from build123d import *

# Parameters (mm, degrees)
CROQUIS1_W              = 111
CROQUIS1_H              = 40
SALIENTE_EXTRUIR1_DEPTH = 5
CROQUIS2_R              = 2
CROQUIS2_W              = 52.7
CROQUIS2_H              = 11.179597985
CORTAR_EXTRUIR1_DEPTH   = 10
CROQUIS3_W              = 5
CROQUIS3_H              = 13.3
SALIENTE_EXTRUIR2_DEPTH = 5
CROQUIS4_W              = 5
CROQUIS4_H              = 13.3
SALIENTE_EXTRUIR3_DEPTH = 5


with BuildPart() as part:
    # Croquis1 → Saliente-Extruir1 (new body)
    with BuildSketch(Plane.XY):
        with Locations((55.5, 20)):
            Rectangle(CROQUIS1_W, CROQUIS1_H)
    extrude(amount=SALIENTE_EXTRUIR1_DEPTH)

    # Croquis2 → Cortar-Extruir1 (cut)
    with BuildSketch(Plane.XY.offset(5)):
        with Locations((24.25, 24.5)):
            Circle(CROQUIS2_R)
        with Locations((86.75, 24.5)):
            Circle(CROQUIS2_R)
        with Locations((24.25, 4.9)):
            Circle(CROQUIS2_R)
        with Locations((86.75, 4.9)):
            Circle(CROQUIS2_R)
        with Locations((54.905498666, 24.410201008)):
            Rectangle(CROQUIS2_W, CROQUIS2_H)
    extrude(amount=-CORTAR_EXTRUIR1_DEPTH, mode=Mode.SUBTRACT)

    # Croquis3 → Saliente-Extruir2 (add)
    with BuildSketch(Plane.ZY):
        with Locations((2.5, 17.85)):
            Rectangle(CROQUIS3_W, CROQUIS3_H)
    extrude(amount=SALIENTE_EXTRUIR2_DEPTH)

    # Croquis4 → Saliente-Extruir3 (add)
    with BuildSketch(Plane(origin=(111, 0, 0), x_dir=(0, 0, -1), z_dir=(1, 0, 0))):
        with Locations((-2.5, 17.85)):
            Rectangle(CROQUIS4_W, CROQUIS4_H)
    extrude(amount=SALIENTE_EXTRUIR3_DEPTH)


solid = part.part
The model under review builds one solid part; all positions refer to its coordinate system, in mm. A direction names the side the tool comes from. Round coordinates to 2 decimals unless told otherwise and drop trailing zeros. Loops run counter-clockwise (first coordinate to the right, second up) from the corner with the lowest first, then second, coordinate; pieces in that order, holes last. Notation, with made-up numbers: (-6, 77) -> (47, 77) arc R21 ccw to (47, 82) -> close; hole circle Ø2 at (64, 70.5). An arc over 180 degrees is marked (long way). One line per question, with ' | ' between items. Start each with the question number.
Item 1: Wall thickness on line 1 along X through (y, z) = (5, 3); line 2 along Y through (x, z) = (24.25, 1.6); line 3 along X through (y, z) = (20, 1.45): over which ranges is each line inside the solid? List them lowest first. Write a range as [from, to].
Item 2: Add section D-D, the plane x = 41. Write out the cut boundary in (y, z), then the cut area to 3 significant figures.
Item 3: For pin 1 (1.5 mm diameter, centred on y = 26, z = 2.5, fed in from +X); pin 2 (1.5 mm diameter, centred on x = 53.5, y = 21.5, fed in from -Z); pin 3 (2.5 mm diameter, centred on y = 31.5, z = 2, fed in from -X); pin 4 (2.5 mm diameter, centred on x = -2, z = 3, fed in from +Y), all flat-tipped, find the tip position at first contact; note any pin that passes through.
Item 4: Add section C-C, the plane z = 3.3. Write out the cut boundary in (x, y).
Item 5: Add section B-B, the plane x = 24.25. Write out the cut boundary in (y, z), then the cut area to 3 significant figures.
Item 6: Draft analysis for pull direction Y (two halves, no side actions). For faces 1 (the face through (116, 18, 3)), 2 (the face through (-2, 11.2, 2)), 3 (the face through (22.663, 23.283, 2.535)), state which applies: +Y half, -Y half, draft (parallel to the pull), parting line (faces both ways), or undercut.
Item 7: Add section A-A, the plane y = 4.9. Write out the cut boundary in (x, z), then the cut area to 3 significant figures.
Item 8: Machinability: for faces 4 (the face through (55, 18.82, 3)), 5 (the face through (113, 11.2, 3)), 6 (the face through (-2, 24.5, 2)), which of the approach directions +Z, -Z, +X, -X, +Y, -Y give a long, thin tool a straight path to every point of the face, cutting with its end or side? Answer none if there is none.
Return value:
1) line 1: x = [0, 22.25], [26.25, 84.75], [88.75, 111] | line 2: y = [0, 2.9], [6.9, 22.5], [26.5, 40] | line 3: x = [-5, 28.56], [81.26, 116]
2) outline: (0, 0) -> (18.82, 0) -> (18.82, 5) -> (0, 5) -> close; (30, 0) -> (40, 0) -> (40, 5) -> (30, 5) -> close | area: 144 mm2
3) pin 1: stops at x = 111 | pin 2: passes through | pin 3: stops at x = 0 | pin 4: stops at y = 24.5
4) outline: (-5, 11.2) -> (0, 11.2) -> (0, 0) -> (111, 0) -> (111, 11.2) -> (116, 11.2) -> (116, 24.5) -> (111, 24.5) -> (111, 40) -> (0, 40) -> (0, 24.5) -> (-5, 24.5) -> close; hole circle Ø4 at (24.25, 4.9); hole circle Ø4 at (24.25, 24.5); hole (28.56, 18.82) -> (81.26, 18.82) -> (81.26, 30) -> (28.56, 30) -> close; hole circle Ø4 at (86.75, 4.9); hole circle Ø4 at (86.75, 24.5)
5) outline: (0, 0) -> (2.9, 0) -> (2.9, 5) -> (0, 5) -> close; (6.9, 0) -> (22.5, 0) -> (22.5, 5) -> (6.9, 5) -> close; (26.5, 0) -> (40, 0) -> (40, 5) -> (26.5, 5) -> close | area: 160 mm2
6) face 1: draft | face 2: -Y half | face 3: undercut
7) outline: (0, 0) -> (22.25, 0) -> (22.25, 5) -> (0, 5) -> close; (26.25, 0) -> (84.75, 0) -> (84.75, 5) -> (26.25, 5) -> close; (88.75, 0) -> (111, 0) -> (111, 5) -> (88.75, 5) -> close | area: 515 mm2
8) face 4: +Z, -Z | face 5: +Z, -Z, +X, -Y | face 6: +Z, -Z, -X, +Y
